from build123d import *

# Parameters (mm, degrees)
SKETCH6_W           = 20
SKETCH6_H           = 16
BOSS_EXTRUDE5_DEPTH = 6
SKETCH7_W           = 10
SKETCH7_H           = 16
BOSS_EXTRUDE6_DEPTH = 3
SKETCH8_W           = 14.5
SKETCH8_H           = 16
BOSS_EXTRUDE7_DEPTH = 13
SKETCH9_R           = 5
CUT_EXTRUDE1_DEPTH  = 32.890437438
FILLET1_R           = 7.5
FILLET2_R           = 7.5


with BuildPart() as part:
    # Sketch6 → Boss-Extrude5 (new body)
    with BuildSketch(Plane(origin=(0, 0, 0), x_dir=(1, 0, 0), z_dir=(0, 1, 0))):
        with Locations((10, 8)):
            Rectangle(SKETCH6_W, SKETCH6_H)
    extrude(amount=BOSS_EXTRUDE5_DEPTH)

    # Sketch7 → Boss-Extrude6 (add)
    with BuildSketch(Plane.XZ):
        with Locations((10, -8)):
            Rectangle(SKETCH7_W, SKETCH7_H)
    extrude(amount=BOSS_EXTRUDE6_DEPTH)

    # Sketch8 → Boss-Extrude7 (add)
    with BuildSketch(Plane(origin=(0, 6, 0), x_dir=(1, 0, 0), z_dir=(0, 1, 0))):
        with Locations((10, 8)):
            Rectangle(SKETCH8_W, SKETCH8_H)
    extrude(amount=BOSS_EXTRUDE7_DEPTH)

    # Sketch9 → Cut-Extrude1 (cut, through all)
    with BuildSketch(Plane.XY):
        with Locations((10, 11)):
            Circle(SKETCH9_R)
    extrude(amount=-CUT_EXTRUDE1_DEPTH, mode=Mode.SUBTRACT)

    # Fillet1
    # the kernel refuses this fillet: 7.5 mm, written as the material it takes off along each edge
    with BuildSketch(Plane(origin=(17.25, 19, -34.75), x_dir=(-1, 0, 0), z_dir=(0, 0, 1))) as fillet1_piece_1:
        with BuildLine():
            CenterArc((FILLET1_R, FILLET1_R), FILLET1_R, 180, 90)
            Line((0, FILLET1_R), (0, 0))
            Line((0, 0), (FILLET1_R, 0))
        make_face()
    extrude(amount=53.5, mode=Mode.SUBTRACT)
    with BuildSketch(Plane(origin=(2.75, 19, 18.75), x_dir=(0, -1, 0), z_dir=(0, 0, -1))) as fillet1_piece_2:
        with BuildLine():
            CenterArc((FILLET1_R, -FILLET1_R), FILLET1_R, 90, 90)
            Line((0, -FILLET1_R), (0, 0))
            Line((0, 0), (FILLET1_R, 0))
        make_face()
    extrude(amount=53.5, mode=Mode.SUBTRACT)

    # Fillet2
    # the kernel refuses this fillet: 7.5 mm, written as the material it adds along each edge
    with BuildSketch(Plane(origin=(17.25, 6, -16), x_dir=(1, 0, 0), z_dir=(0, 0, 1))) as fillet2_piece_1:
        with BuildLine():
            CenterArc((7.496865043, 5.806657581), FILLET2_R, 181.171427285, 49.563032728)
            Line((-0.001567478, 5.65332879), (-0.75141073, 5.637995911))
            ThreePointArc((-0.75141073, 5.637995911), (-0.75, 5.5), (-0.75, 0))
            Line((-0.75, 0), (0, -0.75))
            ThreePointArc((0, -0.75), (1.375, -0.75), (2.275313496, -0.580665758))
            Line((2.275313496, -0.580665758), (2.75, 0))
        make_face()
    extrude(amount=16)
    with BuildSketch(Plane(origin=(2.75, 6, 0), x_dir=(0.00027726642617420565, 0.9999999615616638, 0), z_dir=(0, 0, -1))) as fillet2_piece_2:
        with BuildLine():
            CenterArc((5.804578729, -7.498474746), FILLET2_R, 91.155541089, 49.563032728)
            Line((-0.000762483, -2.749999894), (-0.581296604, -2.275152409))
            ThreePointArc((-0.581296604, -2.275152409), (-0.750381213, -1.374791997), (-0.749999971, 0.00020795))
            Line((-0.749999971, 0.00020795), (0.00020795, 0.749999971))
            ThreePointArc((0.00020795, 0.749999971), (5.500207738, 0.748475006), (5.638204036, 0.749847475))
            Line((5.638204036, 0.749847475), (5.653329008, 0))
        make_face()
    extrude(amount=16)


solid = part.part
Can you work these out from the model? Positions are in its coordinate system, mm. A direction names the side the tool comes from. Give positions to 0.01 mm unless a question says otherwise; leave off trailing zeros. Loops run counter-clockwise (first coordinate to the right, second up) from the corner with the lowest first, then second, coordinate; pieces in that order, holes last. Notation, with made-up numbers: (-7.75, 89.25) - (27.25, 89.25) arc R9 cw to (27.25, 106.25) - close; hole circle Ø1 at (66.25, 4). An arc over 180 degrees is marked (long way). One line per item, written item: value.
(1) On a 3-axis mill with a long thin cutter (end or side, diameter ignored), from which of +Z, -Z, +X, -X, +Y, -Y can I reach the whole of each face in a straight line? I mean faces 4 (the face through (20, 3, -8)), 5 (the face through (17, 0, -8)). Say none if no direction works.
Verdict:
face 4: +Z, -Z, +X, +Y, -Y
face 5: +Z, -Z, +X, -Y
(2) I need wall thicknesses on line 1 along Y through (x, z) = (8.5, -15); line 2 along Y through (x, z) = (10, -6.5); line 3 along X through (y, z) = (-1.5, -11). Which ranges of each line are inside material? Lowest first, please.
Verdict:
line 1: -3 to 6.23, 15.77 to 18.79
line 2: -3 to 6, 16 to 19
line 3: 5 to 15
(3) I'm going to push flat-ended pins straight in: pin 1 (6 mm diameter, centred on y = 9.5, z = -14, fed in from -X); pin 2 (2 mm diameter, centred on y = 16, z = -13, fed in from -X); pin 3 (1.5 mm diameter, centred on x = 2.5, z = -12, fed in from -Y). Where does each tip first touch, or does it pass through?
Verdict:
pin 1: x = 0.55
pin 2: x = 3.62
pin 3: y = 0
(4) If we section it at B-B, the plane y = 11: List the corners of the cut face in (x, z) for me.
Verdict:
outline: (2.71, -16) - (5, -16) - (5, 0) - (2.71, 0) - close; (15, -16) - (17.29, -16) - (17.29, 0) - (15, 0) - close
(5) If we section it at D-D, the plane y = -1.5: List the corners of the cut face in (x, z) for me.
Verdict:
outline: (5, -16) - (15, -16) - (15, 0) - (5, 0) - close
(6) If we mould it in two halves opening along X, with no side actions, what happens to faces 1 (the face through (2, 0, -8)), 2 (the face through (14.77, 12.5, -7.89)), 3 (the face through (5, -1, -8))? For each: released by +X, released by -X, zero draft, split by the parting line, or undercut.
Verdict:
face 1: zero draft
face 2: undercut
face 3: released by -X
(7) If we section it at C-C, the plane x = 6: List the corners of the cut face in (y, z) for me.
Verdict:
outline: (-3, -16) - (8, -16) - (8, 0) - (-3, 0) - close; (14, -16) - (17.68, -16) - (17.68, 0) - (14, 0) - close
(8) If we section it at A-A, the plane z = -4: List the corners of the cut face in (x, y) for me, plus the area to 3 significant figures.
Verdict:
outline: (0, 0) - (5, 0) - (5, -3) - (15, -3) - (15, 0) - (20, 0) - (20, 6) arc R7.5 cw to (17.25, 11.65) arc R7.5 ccw to (10, 19) arc R7.5 ccw to (2.75, 11.65) arc R7.5 cw to (0, 6) - close; hole circle Ø10 at (10, 11)
area: 246 mm^2
